```python
from build123d import *

# Parameters (mm, degrees)
F0_W     = 75.692
F0_H     = 154.686
F1_DEPTH = 8.636
F2_R     = 5.08
F3_SIZE  = 2.54


with BuildPart() as f1:
    # F0 (on Front) → F1 (new body)
    with BuildSketch(Plane.XZ):
        Rectangle(F0_W, F0_H)
    extrude(amount=F1_DEPTH)

    # F2
    f2_edges = [f1.edges().sort_by_distance(p)[0] for p in [
        (37.846, 0, 0),
        (0, 0, 77.343),
        (-37.846, 0, 0),
        (0, 0, -77.343),
    ]]
    fillet(f2_edges, radius=F2_R)

    # F3
    f3_edges = [f1.edges().sort_by_distance(p)[0] for p in [
        (0, -8.636, 77.343),
        (-37.846, -8.636, 0),
        (0, -8.636, -77.343),
        (37.846, -8.636, 0),
    ]]
    chamfer(f3_edges, length=F3_SIZE)


solid = f1.part
```
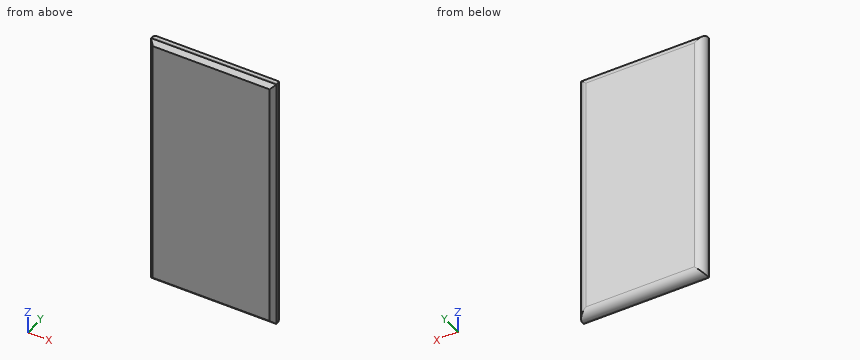
Build history of the part. All positions in model axes, mm. Round coordinates to 2 decimals unless told otherwise and drop trailing zeros. Write each loop counter-clockwise with the first axis right and the second up, starting at its lowest first coordinate (ties: lowest second). Pieces come first, ordered by that corner, then holes.
1) Pin check, flat tip, straight feed: pin 1 (1 mm diameter, centred on x = 27, y = -3, fed in from +Z). Stop position of the tip, or through.
2) Band-saw the part on B-B, the plane y = -2.5. List the corners of the cut face in (x, z), and give its area (3 significant figures).
3) Drill centre lines: probe 1 along Z at (x, y) = (17.5, -4.75); probe 2 along Z at (x, y) = (-23, -1); probe 3 along Y at (x, z) = (34, -68). Where is each one in solid material? Low to high.
4) Band-saw the part on A-A, the plane z = -47. List the corners of the cut face in (x, y).
Ans:
1. pin 1: stops at z = 77.09
2. outline: (-37.14, -76.64) - (37.14, -76.64) - (37.14, 76.64) - (-37.14, 76.64) - close
2. area: 11,400 mm2
3. probe 1: z = -77.33 to 77.33
3. probe 2: z = -75.29 to 75.29
3. probe 3: y = -8.64 to -0.15
4. outline: (-37.85, -6.1) - (-35.31, -8.64) - (35.31, -8.64) - (37.85, -6.1) - (37.85, -5.08) arc R5.08 ccw to (32.77, 0) - (-32.77, 0) arc R5.08 ccw to (-37.85, -5.08) - close
